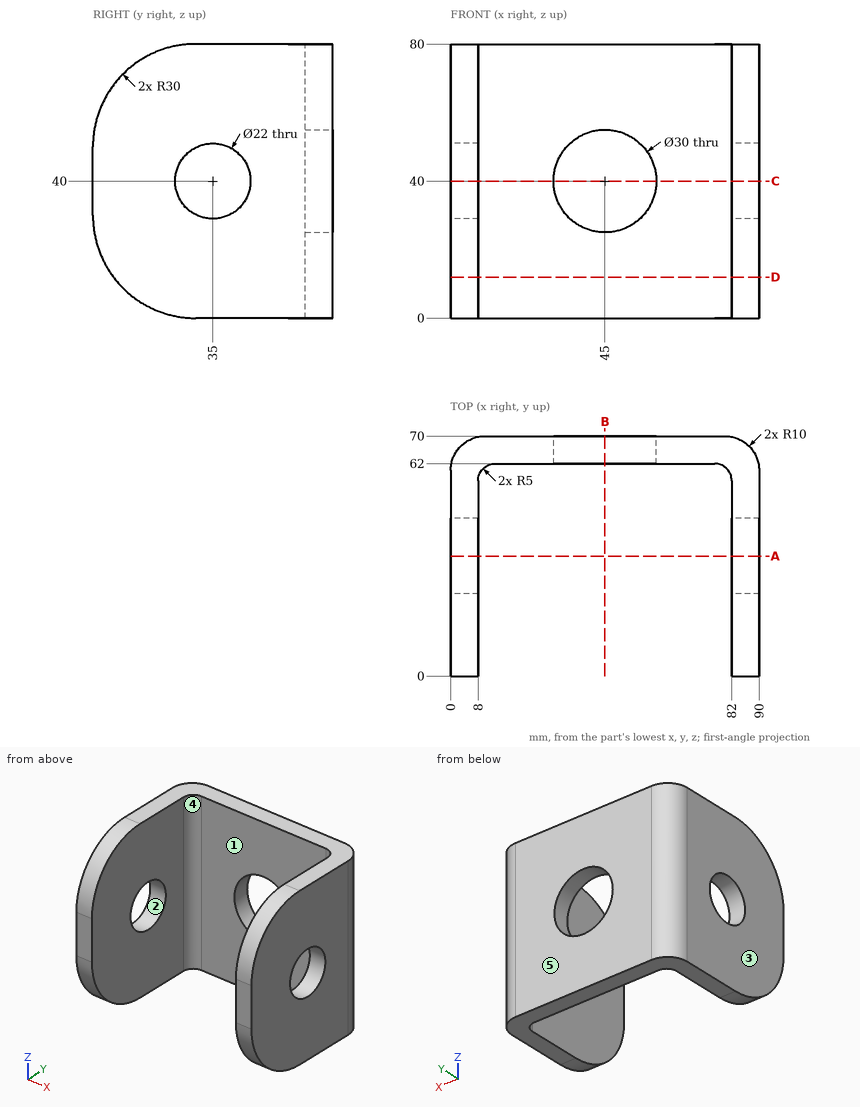
Answer from the drawing. Dimensions are ordinates in mm from the lowest x, y and z of the part. A direction names the side the tool comes from. Coordinates: 2 decimals unless noted, no trailing zeros. Loops run counter-clockwise (first coordinate to the right, second up) from the corner with the lowest first, then second, coordinate; pieces in that order, holes last. Notation, with made-up numbers: (3, 7.25) - (15, 7.25) arc R18 cw to (15, 34.25) - close; hole circle Ø6 at (28.5, 31.25). An arc over 180 degrees is marked (long way). Answer in a Markdown table with one row per item.
1. Find section B-B, the plane x = 45. Write down the section's boundary in (y, z), then the cut area to 3 significant figures.
Conclusion:
| item | result |
|---|---|
| outline | (62, 0) - (70, 0) - (70, 25) - (62, 25) - close; (62, 55) - (70, 55) - (70, 80) - (62, 80) - close |
| area | 400 mm² |
2. Find section D-D, the plane z = 12. Write down the section's boundary in (x, y), then the cut area to 3 significant figures.
Conclusion:
| item | result |
|---|---|
| outline | (0, 6) - (8, 6) - (8, 57) arc R5 cw to (13, 62) - (77, 62) arc R5 cw to (82, 57) - (82, 6) - (90, 6) - (90, 60) arc R10 ccw to (80, 70) - (10, 70) arc R10 ccw to (0, 60) - close |
| area | 1,580 mm² |
3. Determine the mould class of the marked faces 1, 2 and 3 for opening direction X: +X half, -X half, draft (parallel to the pull), parting line (faces both ways), or undercut.
Conclusion:
| item | result |
|---|---|
| face 1 | undercut |
| face 2 | draft |
| face 3 | -X half |
4. Find section C-C, the plane z = 40. Write down the section's boundary in (x, y), then the cut area to 3 significant figures.
Conclusion:
| item | result |
|---|---|
| outline | (0, 0) - (8, 0) - (8, 24) - (0, 24) - close; (0, 46) - (8, 46) - (8, 57) arc R5 cw to (13, 62) - (30, 62) - (30, 70) - (10, 70) arc R10 ccw to (0, 60) - close; (60, 62) - (77, 62) arc R5 cw to (82, 57) - (82, 46) - (90, 46) - (90, 60) arc R10 ccw to (80, 70) - (60, 70) - close; (82, 0) - (90, 0) - (90, 24) - (82, 24) - close |
| area | 1,090 mm² |
5. Given pin 1 (12 mm diameter, centred on y = 16.5, z = 51.5, fed in from -X); pin 2 (3 mm diameter, centred on x = 57.5, z = 18.5, fed in from -Y), each flat-ended and moving along its own axis, determine where each tip first touches the part or whether it passes through.
Conclusion:
| item | result |
|---|---|
| pin 1 | stops at x = 0 |
| pin 2 | stops at y = 62 |
6. Straight lines are drawn through the part: line 1 (X direction, y = 4, z = 30); line 2 (Z direction, x = 85, y = 35); line 3 (Z direction, x = 45, y = 68.75). For each, find the intervals that lie inside material, in ascending order.
Conclusion:
| item | result |
|---|---|
| line 1 | x = 0 to 8, 82 to 90 |
| line 2 | z = 0 to 29, 51 to 80 |
| line 3 | z = 0 to 25, 55 to 80 |
7. Find section A-A, the plane y = 35. Write down the section's boundary in (x, z).
Conclusion:
| item | result |
|---|---|
| outline | (0, 0) - (8, 0) - (8, 29) - (0, 29) - close; (0, 51) - (8, 51) - (8, 80) - (0, 80) - close; (82, 0) - (90, 0) - (90, 29) - (82, 29) - close; (82, 51) - (90, 51) - (90, 80) - (82, 80) - close |
8. Which of the six approach directions +Z, -Z, +X, -X, +Y, -Y give full straight-line access (tool end or side, diameter ignored) to the marked faces 4 and 5?
Conclusion:
| item | result |
|---|---|
| face 4 | +Z, -Z, -Y |
| face 5 | +Z, -Z, +X, -X, +Y |
